Work out the finished part from the listing and answer in its coordinate system (mm). Coordinates: 2 decimals unless noted, no trailing zeros. Order: outer loops, then holes, each group sorted by start corner. A loop starts at its lowest first (then second) coordinate and runs counter-clockwise, first axis right, second up. Notation, with made-up numbers: (53.25, 48) -> (86.25, 48) arc R16 ccw to (86.25, 79) -> close; hole circle Ø3 at (51, 25). An arc over 180 degrees is marked (long way). Use one line per item in the form item = value.
from build123d import *

# Parameters (mm, degrees)
SKETCH_1_R      = 1.5
SKETCH_1_R_2    = 2.5
SKETCH_1_R_3    = 1.55
SKETCH_1_R_4    = 1
EXTRUDE_1_DEPTH = 3


with BuildPart() as part:
    # 草图1 → 凸台-拉伸1 (new body)
    with BuildSketch(Plane(origin=(0, 0, 0), x_dir=(1, 0, 0), z_dir=(0, 1, 0))):
        with BuildLine():
            Line((132, -5), (132, -25))
            ThreePointArc((132, -25), (130.535533906, -28.535533906), (127, -30))
            Line((127, -30), (75, -30))
            ThreePointArc((75, -30), (71.464466094, -28.535533906), (70, -25))
            Line((70, -25), (70, -5))
            ThreePointArc((70, -5), (68.535533906, -1.464466094), (65, 0))
            Line((65, 0), (58, 0))
            ThreePointArc((58, 0), (51.282485579, 2.782485579), (48.5, 9.5))
            Line((48.5, 9.5), (48.5, 93))
            ThreePointArc((48.5, 93), (51.282485579, 99.717514421), (58, 102.5))
            Line((58, 102.5), (65, 102.5))
            ThreePointArc((65, 102.5), (68.535533906, 103.964466094), (70, 107.5))
            Line((70, 107.5), (70, 127.5))
            ThreePointArc((70, 127.5), (71.464466094, 131.035533906), (75, 132.5))
            Line((75, 132.5), (127, 132.5))
            ThreePointArc((127, 132.5), (130.535533906, 131.035533906), (132, 127.5))
            Line((132, 127.5), (132, 107.5))
            ThreePointArc((132, 107.5), (133.464466094, 103.964466094), (137, 102.5))
            Line((137, 102.5), (162, 102.5))
            ThreePointArc((162, 102.5), (169.071067812, 99.571067812), (172, 92.5))
            Line((172, 92.5), (172, 10))
            ThreePointArc((172, 10), (169.071067812, 2.928932188), (162, 0))
            Line((162, 0), (137, 0))
            ThreePointArc((137, 0), (133.464466094, -1.464466094), (132, -5))
        make_face()
        with Locations(Location((96.855482095, 24.5, 0), (0, 0, 270))):
            Circle(SKETCH_1_R, mode=Mode.SUBTRACT)
        with Locations(Location((135.355482095, 24.5, 0), (0, 0, 270))):
            Circle(SKETCH_1_R, mode=Mode.SUBTRACT)
        with Locations(Location((65.477875917, 19.059382071, 0), (0, 0, 270))):
            Circle(SKETCH_1_R_2, mode=Mode.SUBTRACT)
        with Locations(Location((79.074216313, -16.098364995, 0), (0, 0, 270))):
            Circle(SKETCH_1_R_3, mode=Mode.SUBTRACT)
        with Locations(Location((121.803446989, -16.098364995, 0), (0, 0, 270))):
            Circle(SKETCH_1_R_3, mode=Mode.SUBTRACT)
        with Locations(Location((135.355482095, 78, 0), (0, 0, 90))):
            Circle(SKETCH_1_R, mode=Mode.SUBTRACT)
        with Locations(Location((96.855482095, 78, 0), (0, 0, 90))):
            Circle(SKETCH_1_R, mode=Mode.SUBTRACT)
        with Locations(Location((65.477875917, 83.440617929, 0), (0, 0, 90))):
            Circle(SKETCH_1_R_2, mode=Mode.SUBTRACT)
        with Locations(Location((55, 10, 0), (0, 0, 270))):
            Circle(SKETCH_1_R_4, mode=Mode.SUBTRACT)
        with Locations(Location((55, 92.5, 0), (0, 0, 90))):
            Circle(SKETCH_1_R_4, mode=Mode.SUBTRACT)
        with Locations(Location((121.803446989, 118.598364995, 0), (0, 0, 90))):
            Circle(SKETCH_1_R_3, mode=Mode.SUBTRACT)
        with Locations(Location((79.074216313, 118.598364995, 0), (0, 0, 90))):
            Circle(SKETCH_1_R_3, mode=Mode.SUBTRACT)
        with Locations(Location((137, 90.25, 0), (0, 0, 270))):
            Circle(SKETCH_1_R_3, mode=Mode.SUBTRACT)
        with Locations(Location((137, 12.25, 0), (0, 0, 90))):
            Circle(SKETCH_1_R_3, mode=Mode.SUBTRACT)
    extrude(amount=EXTRUDE_1_DEPTH)


solid = part.part
(1) Straight lines are drawn through the part: line 1 along Z through (x, y) = (137, 1.9); line 2 along Z through (x, y) = (64, 1); line 3 along X through (y, z) = (2, -12.25). For each, find the intervals that lie inside material, in ascending order.
Data:
line_1 = -102.5 to -91.8, -88.7 to -13.8, -10.7 to 0
line_2 = -102.5 to -85.46, -81.42 to -21.08, -17.04 to 0
line_3 = 48.5 to 135.45, 138.55 to 172
(2) Section B-B on z = 12.5 is taken. Write down the section's boundary in (x, y), plus the area to 3 significant figures.
Data:
outline = (70, 0) -> (132, 0) -> (132, 3) -> (70, 3) -> close
area = 186 mm²
(3) Each of these flat-tipped pins is pushed along its axis until it touches: P1, Ø3.5, axis at x = 137, z = -12.25, coming from the -Y side; P2, Ø1.5, axis at y = 2, z = -121, coming from the -X side; P3, Ø1.5, axis at x = 60, y = 2, coming from the -Z side; P4, Ø2.5, axis at x = 135.36, z = -78, coming from the -Y side. Where does it stop, or does it pass through?
Data:
P1 = 0
P2 = 70
P3 = -102.5
P4 = through
(4) Section A-A on x = 143.5 is taken. Write down the section's boundary in (y, z).
Data:
outline = (0, -102.5) -> (3, -102.5) -> (3, 0) -> (0, 0) -> close
(5) The mould has two halves that part along Z. Classify faces 1 (the cylindrical face through (123.34, 1.48, 15.9)), 2 (the cylindrical face through (168.99, 1.48, -99.65)), 3 (the cylindrical face through (69, 1, 2)): released by +Z, released by -Z, zero draft, split by the parting line, or undercut.
Data:
face_1 = undercut
face_2 = released by -Z
face_3 = released by +Z
(6) Section C-C on y = 1 is taken. Count the separate pieces of the cut face and the enclosed holes in it, plus the area to 3 significant figures.
Data:
separate_pieces = 1
enclosed_holes = 14
area = 16,200 mm²
